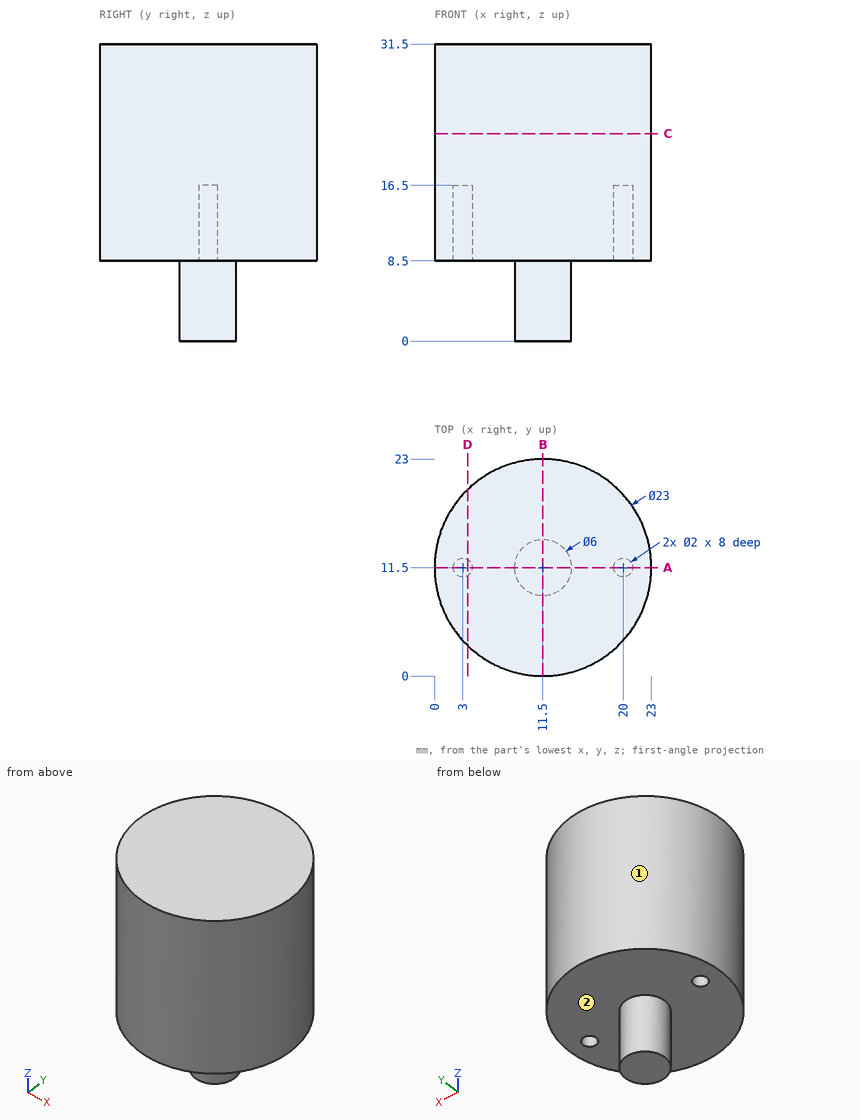
Check sheet for the drawn part. Datum: minimum x, y, z corner. Units: mm. A direction names the side the tool comes from. Round coordinates to 2 decimals unless told otherwise and drop trailing zeros. Write each loop counter-clockwise with the first axis right and the second up, starting at its lowest first coordinate (ties: lowest second). Pieces come first, ordered by that corner, then holes. Notation, with made-up numbers: (-28, 35) -> (-12, 35) arc R22 ccw to (-12, 58) -> close; hole circle Ø4 at (67.25, 30). An arc over 180 degrees is marked (long way). Write each question's results on one line, items separated by ' | '.
Q1. Sectioned sample at A-A, the plane y = 11.5. Record the boundary of the cut face in (x, z).
Derived:
outline: (0, 8.5) -> (2, 8.5) -> (2, 16.5) -> (4, 16.5) -> (4, 8.5) -> (8.5, 8.5) -> (8.5, 0) -> (14.5, 0) -> (14.5, 8.5) -> (19, 8.5) -> (19, 16.5) -> (21, 16.5) -> (21, 8.5) -> (23, 8.5) -> (23, 31.5) -> (0, 31.5) -> close
Q2. Sectioned sample at C-C, the plane z = 22. Record the boundary of the cut face in (x, y), and give its area (3 significant figures).
Derived:
outline: circle Ø23 at (11.5, 11.5) | area: 415 mm²
Q3. Sectioned sample at D-D, the plane x = 3.5. Record the boundary of the cut face in (y, z).
Derived:
outline: (3.24, 8.5) -> (10.63, 8.5) -> (10.63, 16.5) -> (12.37, 16.5) -> (12.37, 8.5) -> (19.76, 8.5) -> (19.76, 31.5) -> (3.24, 31.5) -> close
Q4. Sectioned sample at B-B, the plane x = 11.5. Record the boundary of the cut face in (y, z), and give its area (3 significant figures).
Derived:
outline: (0, 8.5) -> (8.5, 8.5) -> (8.5, 0) -> (14.5, 0) -> (14.5, 8.5) -> (23, 8.5) -> (23, 31.5) -> (0, 31.5) -> close | area: 580 mm²
Q5. Go/stop test with flat-tipped pins: pin 1 Ø12 at (y, z) = (3, 10) entering from +X (3 decimals); pin 2 Ø3 at (y, z) = (18.5, 8) entering from -X; pin 3 Ø1 at (y, z) = (16, 25) entering from -X. Record where each tip stops, or that it passes through.
Derived:
pin 1: stops at x = 22.725 | pin 2: stops at x = 1.45 | pin 3: stops at x = 0.72
Q6. Access from +Z, -Z, +X, -X, +Y, -Y to the whole of each face (thin tool, end or side, straight path). Record for the marked faces 1 and 2.
Derived:
face 1: +Z, -Z | face 2: -Z
Q7. Thickness scan on probe 1 along Z at (x, y) = (14.75, 9.5); probe 2 along Y at (x, z) = (20, 14.25); probe 3 along Z at (x, y) = (20, 11.5). Record the ranges inside material, lowest first.
Derived:
probe 1: z = 8.5 to 31.5 | probe 2: y = 3.75 to 10.5, 12.5 to 19.25 | probe 3: z = 16.5 to 31.5
